Work out the finished part from the listing and answer in its coordinate system (mm). A direction names the side the tool comes from. Give positions to 0.01 mm unless a question says otherwise; leave off trailing zeros. Loops run counter-clockwise (first coordinate to the right, second up) from the corner with the lowest first, then second, coordinate; pieces in that order, holes last. Notation, with made-up numbers: (45.5, 23) - (79.5, 23) arc R15 cw to (79.5, 40) - close; hole circle Ø11 at (-11.5, 85). An arc over 180 degrees is marked (long way). One line per question, with ' | ' between items. Start each with the question number.
1. Which of the six approach directions +Z, -Z, +X, -X, +Y, -Y give full straight-line access (tool end or side, diameter ignored) to faces 1 (the face through (3.66, 28, -10)), 2 (the face through (-0.467, -14, 2)), 3 (the face through (15, 26.298, -10))?
2. Find the intervals of material crossed by line 1 (Y direction, x = -7.5, z = 1.25); line 2 (Y direction, x = -10, z = 0.5); line 3 (Y direction, x = 6, z = 1.25), in increasing order.
3. Section B-B (x = 1.5) is taken. Determine the outline of the cut face in (y, z) (3 decimals), plus the area to 3 significant figures.
4. Each of these flat-tipped pins is pushed along its axis until it touches: pin 1 (3 mm diameter, centred on x = 2.5, y = 7.5, fed in from +Z); pin 2 (2.5 mm diameter, centred on y = -24.5, z = 1.5, fed in from +X); pin 3 (1 mm diameter, centred on x = -9, y = 28, fed in from -Z); pin 4 (4 mm diameter, centred on x = 3.5, z = -9.5, fed in from -Y). Where does it stop, or does it pass through?
5. Section A-A (z = -5) is taken. Determine the outline of the cut face in (x, y).
6. Section C-C (x = -7) is taken. Determine the outline of the cut face in (y, z) (3 decimals), plus the area to 3 significant figures.
7. Section D-D (y = 6.5) is taken. Determine the outline of the cut face in (x, z) (3 decimals).
8. For a pull along X with two mould halves and no side action, classify faces 4 (the face through (4, 23.123, -1)), 5 (the face through (-7.23, -10.88, 1.57)), 6 (the face through (-16.342, -1, 1)) as released by +X, released by -X, zero draft, split by the parting line, or undercut.
from build123d import *

# Parameters (mm, degrees)
SKETCH1_W           = 15.875
SKETCH1_H           = 79.375
SKETCH1_R           = 2.54
BOSS_EXTRUDE1_DEPTH = 3.175
BOSS_EXTRUDE2_DEPTH = 3.175
SKETCH3_W           = 17.4625
SKETCH3_H           = 3.175
BOSS_EXTRUDE3_DEPTH = 3.175


with BuildPart() as part:
    # Sketch1 → Boss-Extrude1 (new body)
    with BuildSketch(Plane.XY):
        with Locations((-8.404682644, -10.214522003)):
            Rectangle(SKETCH1_W, SKETCH1_H)
        with Locations((-8.404682644, -8.627022003)):
            Circle(SKETCH1_R, mode=Mode.SUBTRACT)
        with Locations((-8.404682644, -40.377022003)):
            Circle(SKETCH1_R, mode=Mode.SUBTRACT)
    extrude(amount=BOSS_EXTRUDE1_DEPTH)

    # Sketch2 → Boss-Extrude2 (add)
    with BuildSketch(Plane(origin=(0, 29.472977997, 0), x_dir=(1, 0, 0), z_dir=(0, 1, 0))):
        Polygon((-0.467182644, 0), (3.660317356, 0), (3.660317356, 3.175), (3.660317356, 16.51), (-16.342182644, 16.51), (-16.342182644, 0), align=None)
        Polygon((16.995317356, 0), (3.660317356, 0), (-0.467182644, 0), (-0.467182644, -3.175), (16.995317356, -3.175), align=None)
        Polygon((3.660317356, 3.175), (3.660317356, 0), (16.995317356, 0), (16.995317356, 16.531210472), (13.820317356, 16.531210472), (13.820317356, 3.175), align=None)
    extrude(amount=-BOSS_EXTRUDE2_DEPTH)

    # Sketch3 → Boss-Extrude3 (add)
    with BuildSketch(Plane.XZ.offset(-26.297977997)):
        Polygon((-0.467182644, 0), (-16.342182644, 0), (-16.342182644, -3.175), (3.660317356, -3.175), (13.820317356, -3.175), (16.995317356, -3.175), (16.995317356, 0), align=None)
        with Locations((8.264067356, 1.5875)):
            Rectangle(SKETCH3_W, SKETCH3_H)
    extrude(amount=BOSS_EXTRUDE3_DEPTH)


solid = part.part
Conclusion:
1) face 1: -Z, +Y, -Y | face 2: +Z, -Z, +X, -Y | face 3: -Z, +X, -X, -Y
2) line 1: -49.9 to -42.75, -38 to -11, -6.25 to 29.47 | line 2: -49.9 to -42.35, -38.4 to -10.6, -6.65 to 29.47 | line 3: 23.12 to 29.47
3) outline: (23.123, -3.175) - (26.298, -3.175) - (26.298, -16.51) - (29.473, -16.51) - (29.473, 3.175) - (23.123, 3.175) - close | area: 82.7 mm²
4) pin 1: through | pin 2: x = -0.47 | pin 3: z = -16.51 | pin 4: y = 26.3
5) outline: (-16.34, 26.3) - (3.66, 26.3) - (3.66, 29.47) - (-16.34, 29.47) - close; (13.82, 26.3) - (17, 26.3) - (17, 29.47) - (13.82, 29.47) - close
6) outline: (-49.902, 0) - (-42.493, 0) - (-42.493, 3.175) - (-49.902, 3.175) - close; (-38.261, 0) - (-10.743, 0) - (-10.743, 3.175) - (-38.261, 3.175) - close; (-6.511, 0) - (23.123, 0) - (23.123, -3.175) - (26.298, -3.175) - (26.298, -16.51) - (29.473, -16.51) - (29.473, 3.175) - (-6.511, 3.175) - close | area: 288 mm²
7) outline: (-16.342, 0) - (-0.467, 0) - (-0.467, 3.175) - (-16.342, 3.175) - close
8) face 4: zero draft | face 5: undercut | face 6: released by -X
